Build history of the part. All positions in model axes, mm. Give positions to 0.01 mm unless a question says otherwise; leave off trailing zeros. Write each loop counter-clockwise with the first axis right and the second up, starting at its lowest first coordinate (ties: lowest second). Pieces come first, ordered by that corner, then holes. Notation, with made-up numbers: (33.25, 38) -> (85.25, 38) arc R26 ccw to (85.25, 58) -> close; hole circle Ø2 at (14, 69.5). An arc over 180 degrees is marked (long way). One line per question, with ' | ' between items. Start each with the question number.
(1) Drill centre lines: probe 1 along Y at (x, z) = (0, 20) (1 decimal); probe 2 along X at (y, z) = (2.25, 36); probe 3 along Y at (x, z) = (-1.75, 16). Where is each one in solid material? Low to high. Write a range as from..to.
(2) Band-saw the part on B-B, the plane z = 68.5. Give the cut face in (x, y) (1 decimal).
(3) Pull direction X, two halves, no side cores. Call faces 1 (the cylindrical face through (-3.78, -2.9, 37.57)), 2 (the cylindrical face through (-0.69, 3.1, 32.87)): released by +X, released by -X, zero draft, split by the parting line, or undercut.
(4) Pin check, flat tips, straight feed: P1, Ø4, axis at x = 2.5, z = 26, coming from the +Y side; P2, Ø5.5, axis at x = 0, y = 0, coming from the +Z side; P3, Ø2, axis at y = -3.5, z = 52, coming from the -X side. Stop position of each tip, or through.
from build123d import *

# Parameters (mm, degrees)
F0_R     = 4.7625
F1_DEPTH = 76.2
F2_R     = 3.175
F3_DEPTH = 3.175
F4_R     = 3.17499
F5_R     = 3.175
F6_DEPTH = 69.85
F7_R     = 3.175


# Not quite as in the source:
# - a fillet or chamfer is up to 0.001 mm smaller than in the source, because OpenCascade refuses the exact size


with BuildPart() as f1:
    # F0 (on Top) → F1 (new body)
    with BuildSketch(Plane.XY):
        Circle(F0_R)
    extrude(amount=F1_DEPTH)

    # F2 (on face) → F3 (cut)
    with BuildSketch(Plane.XY.offset(76.2)):
        Circle(F2_R)
    extrude(amount=-F3_DEPTH, mode=Mode.SUBTRACT)

    # F4 (radius 3.175 in the source; OpenCascade refuses exactly that, so slightly less here)
    f4_edges = [f1.edges().sort_by_distance(p)[0] for p in [
        (-3.175, 0, 73.025),
    ]]
    fillet(f4_edges, radius=F4_R)

    # F5 (on face) → F6 (cut)
    with BuildSketch(Plane(origin=(0, 0, 0), x_dir=(1, 0, 0), z_dir=(0, 0, -1))):
        Circle(F5_R)
    extrude(amount=-F6_DEPTH, mode=Mode.SUBTRACT)

    # F7
    f7_edges = [f1.edges().sort_by_distance(p)[0] for p in [
        (-3.175, 0, 69.85),
    ]]
    fillet(f7_edges, radius=F7_R)


solid = f1.part
Results:
1) probe 1: y = -4.8..-3.2, 3.2..4.8 | probe 2: x = -4.2..-2.24, 2.24..4.2 | probe 3: y = -4.43..-2.65, 2.65..4.43
2) outline: circle Ø9.5 at (0, 0); hole circle Ø5.2 at (0, 0)
3) face 1: split by the parting line | face 2: undercut
4) P1: stops at y = 4.74 | P2: stops at z = 74.61 | P3: stops at x = -4.05
